The model under review builds one solid part; all positions refer to its coordinate system, in mm. A direction names the side the tool comes from. Round coordinates to 2 decimals unless told otherwise and drop trailing zeros. Write each loop counter-clockwise with the first axis right and the second up, starting at its lowest first coordinate (ties: lowest second). Pieces come first, ordered by that corner, then holes. Notation, with made-up numbers: M -10,-12.75 L 28,-12.75 A8 cw 28,0.25 Z; hole C 35,27 d9. An arc over 180 degrees is marked long. Write item = value, one per line. Start each with the question number.
Item 1: For pin 1 Ø1 at (x, y) = (12, -77) entering from -Z (3 decimals); pin 2 Ø3 at (x, y) = (40.5, 162.5) entering from +Z (3 decimals); pin 3 Ø20.5 at (x, y) = (34, 68.5) entering from +Z, all flat-tipped, find the tip position at first contact; note any pin that passes through.
Item 2: To check wall thickness, follow line 1 along Y through (x, z) = (-6.5, -95.5); line 2 along Y through (x, z) = (-1.5, -30); line 3 along Y through (x, z) = (-6.5, -26). State the ranges of each line that lie inside material, in increasing order.
Item 3: The part is to be moulded in two halves that separate along X. For faces 4 (the flat face through (1, -255.588, -235)), 5 (the flat face through (-101.6, 1, -4)), 6 (the cylindrical face through (95.72, -246.04, -234.79)), 7 (the cylindrical face through (-95.72, 246.04, -457.4)), say which applies: +X half, -X half, draft (parallel to the pull), parting line (faces both ways), or undercut.
Item 4: Take a section at C-C, the plane y = 50. Give the boundary of the cut face in (x, z) (3 decimals), plus the area to 3 significant figures.
Item 5: Tool access review of faces 1 (the flat face through (24, 18.914, -17)), 2 (the cylindrical face through (-93.45, -243.82, -234.79)), 3 (the cylindrical face through (-102.3, 227.5, -38.7)): name each direction out of +Z, -Z, +X, -X, +Y, -Y from which nothing blocks a thin tool from reaching the whole face with its end or side.
Item 6: Take a section at A-A, the plane x = -63. Give the number of separate pieces and of enclosed holes in the cut face, plus the area to 3 significant figures.
from build123d import *

# Parameters (mm, degrees)
EXTRUDE1_DEPTH     = 476.25
CUT_EXTRUDE1_DEPTH = 210.55
EXTRUDE2_DEPTH     = 203.2
SKETCH5_W          = 105.681165702
SKETCH5_H          = 68.064456382
CUT_EXTRUDE2_DEPTH = 15.875


with BuildPart() as part:
    # Sketch1 → Extrude1 (new body)
    with BuildSketch(Plane.XY):
        with BuildLine():
            Line((-73.025, 255.5875), (73.025, 255.5875))
            ThreePointArc((73.025, 255.5875), (95.475640303, 246.288140303), (104.775, 223.8375))
            Line((104.775, 223.8375), (104.775, -223.8375))
            ThreePointArc((104.775, -223.8375), (95.475640303, -246.288140303), (73.025, -255.5875))
            Line((73.025, -255.5875), (-73.025, -255.5875))
            ThreePointArc((-73.025, -255.5875), (-95.475640303, -246.288140303), (-104.775, -223.8375))
            Line((-104.775, -223.8375), (-104.775, 223.8375))
            ThreePointArc((-104.775, 223.8375), (-95.475640303, 246.288140303), (-73.025, 255.5875))
        make_face()
        with BuildLine():
            Line((-101.6, 223.8375), (-101.6, -223.8375))
            ThreePointArc((-101.6, -223.8375), (-93.230576272, -244.043076272), (-73.025, -252.4125))
            Line((-73.025, -252.4125), (73.025, -252.4125))
            ThreePointArc((73.025, -252.4125), (93.230576272, -244.043076272), (101.6, -223.8375))
            Line((101.6, -223.8375), (101.6, 223.8375))
            ThreePointArc((101.6, 223.8375), (93.230576272, 244.043076272), (73.025, 252.4125))
            Line((73.025, 252.4125), (-73.025, 252.4125))
            ThreePointArc((-73.025, 252.4125), (-93.230576272, 244.043076272), (-101.6, 223.8375))
        make_face(mode=Mode.SUBTRACT)
    extrude(amount=-EXTRUDE1_DEPTH)

    # Sketch2 → Cut-Extrude1 (cut, through all)
    with BuildSketch(Plane(origin=(104.775, 0, 0), x_dir=(0, 0, -1), z_dir=(1, 0, 0))):
        with BuildLine():
            Line((34.925, 236.5375), (34.925, 258.595805141))
            Line((34.925, 258.595805141), (441.325, 258.595805141))
            Line((441.325, 258.595805141), (441.325, 236.5375))
            ThreePointArc((441.325, 236.5375), (437.605256121, 227.557243879), (428.625, 223.8375))
            Line((428.625, 223.8375), (47.625, 223.8375))
            ThreePointArc((47.625, 223.8375), (38.644743879, 227.557243879), (34.925, 236.5375))
        make_face()
    extrude(amount=-CUT_EXTRUDE1_DEPTH, mode=Mode.SUBTRACT)

    # Sketch4 → Extrude2 (add)
    with BuildSketch(Plane(origin=(-101.6, 0, 0), x_dir=(0, 0, -1), z_dir=(1, 0, 0))):
        with BuildLine():
            Line((9.525, 198.4375), (9.525, -198.4375))
            ThreePointArc((9.525, -198.4375), (16.964487758, -216.398012242), (34.925, -223.8375))
            Line((34.925, -223.8375), (441.325, -223.8375))
            ThreePointArc((441.325, -223.8375), (459.285512242, -216.398012242), (466.725, -198.4375))
            Line((466.725, -198.4375), (466.725, 198.4375))
            ThreePointArc((466.725, 198.4375), (459.285512242, 216.398012242), (441.325, 223.8375))
            Line((441.325, 223.8375), (34.925, 223.8375))
            ThreePointArc((34.925, 223.8375), (16.964487758, 216.398012242), (9.525, 198.4375))
        make_face()
    extrude(amount=EXTRUDE2_DEPTH)

    # Sketch5 → Cut-Extrude2 (cut)
    with BuildSketch(Plane.XY.offset(-9.525)):
        with Locations((25.113927792, 52.946208207)):
            Rectangle(SKETCH5_W, SKETCH5_H)
    extrude(amount=-CUT_EXTRUDE2_DEPTH, mode=Mode.SUBTRACT)


solid = part.part
Response values:
q1.pin_1 = -466.725
q1.pin_2 = -9.525
q1.pin_3 = -25.4
q2.line_1 = -255.59 to -252.41, -223.84 to 223.84
q2.line_2 = -255.59 to -252.41, -223.36 to 223.36, 252.41 to 255.59
q2.line_3 = -255.59 to -252.41, -222.22 to 222.22, 252.41 to 255.59
q3.face_4 = draft
q3.face_5 = undercut
q3.face_6 = +X half
q3.face_7 = -X half
q4.outline = M -104.775,-476.25 L -101.6,-476.25 L -101.6,-466.725 L 101.6,-466.725 L 101.6,-476.25 L 104.775,-476.25 L 104.775,0 L 101.6,0 L 101.6,-9.525 L 77.955,-9.525 L 77.955,-25.4 L -27.727,-25.4 L -27.727,-9.525 L -101.6,-9.525 L -101.6,0 L -104.775,0 Z
q4.area = 94,200 mm2
q5.face_1 = +Z
q5.face_2 = +Z, -Z
q5.face_3 = +X, -X, +Y
q6.separate_pieces = 4
q6.enclosed_holes = 0
q6.area = 206,000 mm2
